Can you work these out from the model? Positions are in its coordinate system, mm. A direction names the side the tool comes from. Give positions to 0.01 mm unless a question says otherwise; leave off trailing zeros. Write each loop counter-clockwise with the first axis right and the second up, starting at its lowest first coordinate (ties: lowest second). Pieces come first, ordered by that corner, then holes.
from build123d import *
from OCP.BRepFilletAPI import BRepFilletAPI_MakeChamfer

# Parameters (mm, degrees)
SKIZZE1_W                       = 160
SKIZZE1_H                       = 160
AUFSATZ_LINEAR_AUSTRAGEN1_DEPTH = 10
SKIZZE2_W                       = 170
SKIZZE2_H                       = 170
AUFSATZ_LINEAR_AUSTRAGEN2_DEPTH = 20
FASE1_SIZE                      = 12
FASE1_SIZE2                     = 5
VERRUNDUNG1_R                   = 8
VERRUNDUNG2_R                   = 4


with BuildPart() as part:
    # Skizze1 → Aufsatz-Linear austragen1 (new body)
    with BuildSketch(Plane.XY):
        Rectangle(SKIZZE1_W, SKIZZE1_H)
    extrude(amount=AUFSATZ_LINEAR_AUSTRAGEN1_DEPTH)

    # Skizze2 → Aufsatz-Linear austragen2 (add)
    with BuildSketch(Plane.XY.offset(10)):
        Rectangle(SKIZZE2_W, SKIZZE2_H)
    extrude(amount=AUFSATZ_LINEAR_AUSTRAGEN2_DEPTH)

    # Fase1: one chamfer whose edges measure the first distance from different faces: ONE call of the kernel's chamfer builder (chamfer() names one face for all edges)
    fase1_edges_1 = [part.edges().sort_by_distance(p)[0] for p in [
        (85, 0, 30),
    ]]
    fase1_side_1 = [part.faces().sort_by_distance(p)[0] for p in [
        (85, 0, 20),
    ]]
    fase1_edges_2 = [part.edges().sort_by_distance(p)[0] for p in [
        (0, 85, 30),
    ]]
    fase1_side_2 = [part.faces().sort_by_distance(p)[0] for p in [
        (0, 85, 20),
    ]]
    fase1_edges_3 = [part.edges().sort_by_distance(p)[0] for p in [
        (-85, 0, 30),
    ]]
    fase1_side_3 = [part.faces().sort_by_distance(p)[0] for p in [
        (-85, 0, 20),
    ]]
    fase1_edges_4 = [part.edges().sort_by_distance(p)[0] for p in [
        (0, -85, 30),
    ]]
    fase1_side_4 = [part.faces().sort_by_distance(p)[0] for p in [
        (0, -85, 20),
    ]]
    fase1 = BRepFilletAPI_MakeChamfer(part.part.solid().wrapped)
    for e in fase1_edges_1:
        fase1.Add(FASE1_SIZE, FASE1_SIZE2, e.wrapped, fase1_side_1[0].wrapped)  # the first distance lies on this face
    for e in fase1_edges_2:
        fase1.Add(FASE1_SIZE, FASE1_SIZE2, e.wrapped, fase1_side_2[0].wrapped)  # the first distance lies on this face
    for e in fase1_edges_3:
        fase1.Add(FASE1_SIZE, FASE1_SIZE2, e.wrapped, fase1_side_3[0].wrapped)  # the first distance lies on this face
    for e in fase1_edges_4:
        fase1.Add(FASE1_SIZE, FASE1_SIZE2, e.wrapped, fase1_side_4[0].wrapped)  # the first distance lies on this face
    add(Compound.cast(fase1.Shape()), mode=Mode.REPLACE)

    # Verrundung1
    # the kernel refuses this fillet: 8 mm, written as the material it takes off along each edge
    with BuildSketch(Plane(origin=(85, 85, -10), x_dir=(0, -1, 0), z_dir=(0, 0, 1)), Plane(origin=(85, -85, -10), x_dir=(-1, 0, 0), z_dir=(0, 0, 1))) as verrundung1_piece_1:
        with BuildLine():
            CenterArc((VERRUNDUNG1_R, -VERRUNDUNG1_R), VERRUNDUNG1_R, 90, 90)
            Line((0, -VERRUNDUNG1_R), (0, 0))
            Line((0, 0), (VERRUNDUNG1_R, 0))
        make_face()
    extrude(amount=48, mode=Mode.SUBTRACT)
    with BuildSketch(Plane(origin=(-85, -85, -10), x_dir=(1, 0, 0), z_dir=(0, 0, 1)), Plane(origin=(-85, 85, -10), x_dir=(0, -1, 0), z_dir=(0, 0, 1))) as verrundung1_piece_2:
        with BuildLine():
            CenterArc((VERRUNDUNG1_R, VERRUNDUNG1_R), VERRUNDUNG1_R, 180, 90)
            Line((0, VERRUNDUNG1_R), (0, 0))
            Line((0, 0), (VERRUNDUNG1_R, 0))
        make_face()
    extrude(amount=48, mode=Mode.SUBTRACT)
    with BuildSketch(Plane(origin=(-91.18556701, -91.18556701, 3.154639175), x_dir=(0.9333456062030596, -0.13806887665725864, -0.331365303977417), z_dir=(0.358979079308869, 0.35897907930886913, 0.8615497903412858)), Plane(origin=(-91.18556701, 91.18556701, 3.154639175), x_dir=(-0.13806887665725653, -0.9333456062030596, -0.3313653039774179), z_dir=(0.35897907930886913, -0.358979079308869, 0.8615497903412858))) as verrundung1_piece_3:
        with BuildLine():
            CenterArc((VERRUNDUNG1_R * 0.861549790341, VERRUNDUNG1_R), VERRUNDUNG1_R, 188.506927756, 81.493072244)
            Line((-VERRUNDUNG1_R * 0.127448193837, VERRUNDUNG1_R * 0.852071005917), (0, 0))
            Line((0, 0), (VERRUNDUNG1_R * 0.861549790341, 0))
        make_face()
    extrude(amount=48.390379891, mode=Mode.SUBTRACT)
    with BuildSketch(Plane(origin=(91.18556701, -91.18556701, 3.154639175), x_dir=(-0.9333456062030596, -0.13806887665725678, -0.331365303977418), z_dir=(-0.35897907930886913, 0.358979079308869, 0.8615497903412858)), Plane(origin=(91.18556701, 91.18556701, 3.154639175), x_dir=(0.13806887665725714, -0.9333456062030596, -0.33136530397741776), z_dir=(-0.358979079308869, -0.35897907930886913, 0.8615497903412858))) as verrundung1_piece_4:
        with BuildLine():
            CenterArc((VERRUNDUNG1_R * 0.861549790341, -VERRUNDUNG1_R), VERRUNDUNG1_R, 90, 81.493072244)
            Line((-VERRUNDUNG1_R * 0.127448193837, -VERRUNDUNG1_R * 0.852071005917), (0, 0))
            Line((0, 0), (VERRUNDUNG1_R * 0.861549790341, 0))
        make_face()
    extrude(amount=48.390379891, mode=Mode.SUBTRACT)

    # Verrundung2
    verrundung2_edges = [part.edges().sort_by_distance(p)[0] for p in [
        (80, -80, 5),
        (-80, -80, 5),
        (-80, 80, 5),
        (80, 80, 5),
    ]]
    fillet(verrundung2_edges, radius=VERRUNDUNG2_R)


solid = part.part
(1) For faces 1 (the face through (78.797, -78.859, 5.07)), 2 (the face through (78.859, 78.797, 5.07)), 3 (the face through (80, -1, 5)), which set-ups out of +Z, -Z, +X, -X, +Y, -Y let a thin tool reach every point of the face, with its end or its side?
Returned:
face 1: -Z, +X, -Y
face 2: -Z, +X, +Y
face 3: -Z, +X, +Y, -Y
(2) If I drill on L1, parallel to X at y = -8, z = 2; L2, parallel to Y at x = 34, z = 21, over which ranges is the centre line in solid material (lowest first)?
Returned:
L1: x = -80 to 80
L2: y = -83.75 to 83.75
(3) Will these pins go through, and if not, where does the flat tip stop? P1, Ø4, axis at x = -54.5, z = 23, coming from the +Y side; P2, Ø5, axis at x = 8.5, z = 7, coming from the +Y side; P3, Ø4, axis at y = 17, z = 4, coming from the -X side.
Returned:
P1: stops at y = 83.75
P2: stops at y = 80
P3: stops at x = -80
(4) Imagine slicing it at A-A, the plane y = 33.5. Write out the boundary of the cut face in (x, z), plus the area to 3 significant figures.
Returned:
outline: (-85, 10) - (-80, 10) - (-80, 0) - (80, 0) - (80, 10) - (85, 10) - (85, 18) - (80, 30) - (-80, 30) - (-85, 18) - close
area: 4,940 mm2
